Print and shaded views of the part. All mm, measured from the part's lowest x, y and z. A direction names the side the tool comes from. Coordinates: 2 decimals unless noted, no trailing zeros. Order: outer loops, then holes, each group sorted by start corner. A loop starts at its lowest first (then second) coordinate and runs counter-clockwise, first axis right, second up.
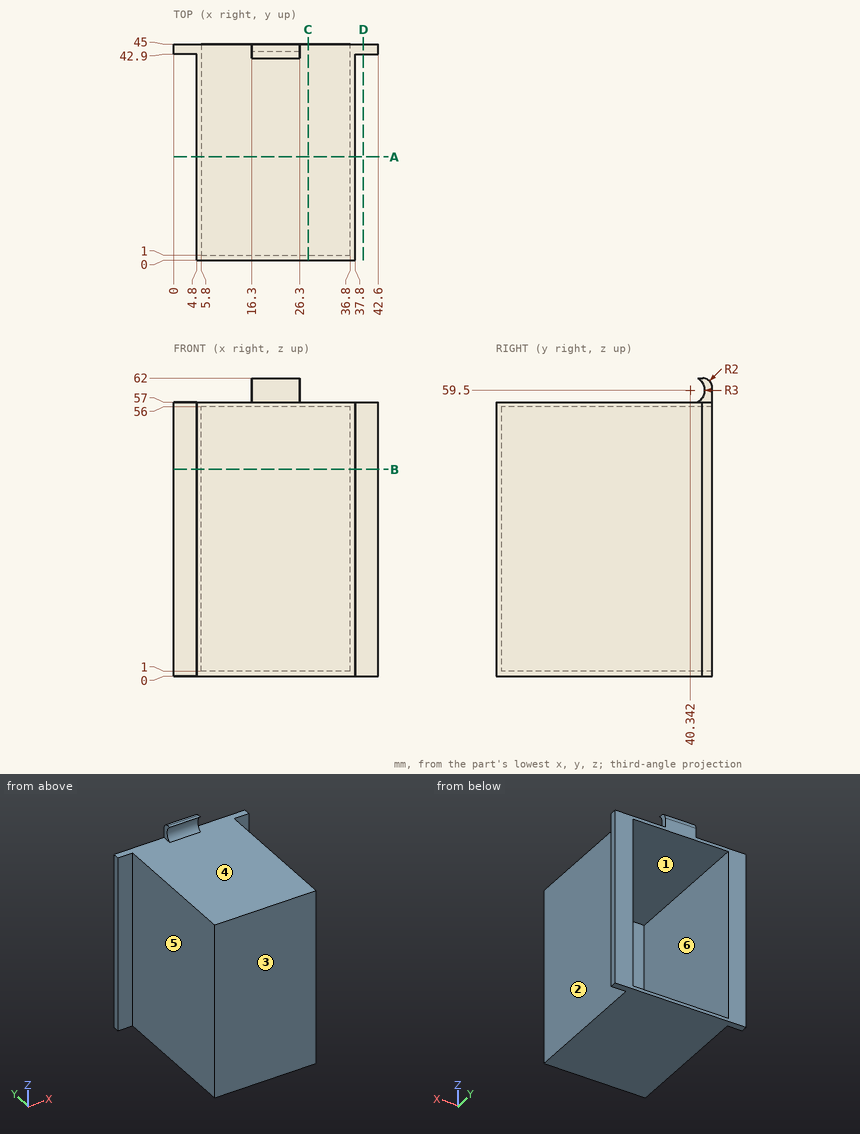
Q1. Cut at A-A, the plane y = 21.5. List the corners of the cut face in (x, z).
Established:
outline: (4.8, 0) - (37.8, 0) - (37.8, 57) - (4.8, 57) - close; hole (5.8, 1) - (36.8, 1) - (36.8, 56) - (5.8, 56) - close
Q2. Which spindle directions (+Z, -Z, +X, -X, +Y, -Y) get a long thin tool onto all of the face, cutting with end or side? Do the marked faces 1, 2 and 3. Say none if no direction does.
Established:
face 1: +Y
face 2: +Z, -Z, +X, -Y
face 3: +Z, -Z, +X, -X, -Y
Q3. Drop flat-ended pins along their axis: P1, Ø15.5, axis at x = 15.5, y = 18, coming from the +Z side; P2, Ø21.5, axis at y = 24, z = 17.5, coming from the -X side; P3, Ø8, axis at y = 19.5, z = 27, coming from the +X side; P4, Ø2, axis at x = 13.5, y = 13.5, coming from the -Z side. Give the stop position or say it passes through.
Established:
P1: stops at z = 57
P2: stops at x = 4.8
P3: stops at x = 37.8
P4: stops at z = 0
Q4. Mould opens along X. For the marked faces 4, 5 and 6 say: pulls with the +X half, pulls with the -X half, needs draft (parallel to the pull), parting line crosses it, or undercut.
Established:
face 4: needs draft
face 5: pulls with the -X half
face 6: undercut
Q5. Cut at B-B, the plane z = 43. List the corners of the cut face in (x, y), plus the area to 3 significant figures.
Established:
outline: (0, 42.9) - (4.8, 42.9) - (4.8, 0) - (37.8, 0) - (37.8, 42.9) - (42.6, 42.9) - (42.6, 45) - (36.8, 45) - (36.8, 1) - (5.8, 1) - (5.8, 45) - (0, 45) - close
area: 141 mm2
Q6. Probe line 1 (Z direction, x = 18, y = 22.5); line 2 (X direction, y = 21.5, z = 29.5); line 3 (Y direction, x = 10, z = 13). List the from-to ranges inside material, lowest first.
Established:
line 1: z = 0 to 1, 56 to 57
line 2: x = 4.8 to 5.8, 36.8 to 37.8
line 3: y = 0 to 1
Q7. Cut at C-C, the plane x = 28. List the corners of the cut face in (y, z), plus the area to 3 significant figures.
Established:
outline: (0, 0) - (45, 0) - (45, 1) - (1, 1) - (1, 56) - (45, 56) - (45, 57) - (0, 57) - close
area: 145 mm2
Q8. Cut at D-D, the plane x = 39.5. List the corners of the cut face in (y, z), plus the area to 3 significant figures.
Established:
outline: (42.9, 0) - (45, 0) - (45, 57) - (42.9, 57) - close
area: 120 mm2
